Source: CAD feature listing. Evaluate the final solid. Frame: model axes, mm. A direction names the side the tool comes from. Give positions to 0.01 mm unless a question says otherwise; leave off trailing zeros. Loops run counter-clockwise (first coordinate to the right, second up) from the corner with the lowest first, then second, coordinate; pieces in that order, holes last.
```python
from build123d import *

# Parameters (mm, degrees)
SKETCH1_R                = 2.1844
BOSS_EXTRUDE1_DEPTH      = 2
SKETCH1_3_W              = 47.380920583
SKETCH1_3_H              = 2
BOSS_EXTRUDE2_DEPTH      = 2
BOSS_EXTRUDE2_DEPTH_BACK = 122.9409
SKETCH2_R                = 3
SKETCH2_W                = 47.380920583
SKETCH2_H                = 2
SKETCH2_R_2              = 2.5
BOSS_EXTRUDE3_DEPTH      = 2
SKETCH2_3_R              = 3
SKETCH2_3_R_2            = 2.5
BOSS_EXTRUDE4_DEPTH      = 1
SKETCH2_4_R              = 2.5
BOSS_EXTRUDE5_DEPTH      = 6
CHAMFER1_SIZE            = 0.5
SKETCH3_R                = 4.5
SKETCH3_R_2              = 1
CUT_EXTRUDE1_DEPTH       = 10
BOSS_EXTRUDE6_DEPTH      = 8.99804


with BuildPart() as part:
    # Sketch1 → Boss-Extrude1 (new body)
    with BuildSketch(Plane(origin=(0, 0, 0), x_dir=(1, 0, 0), z_dir=(0, 1, 0))):
        with BuildLine():
            ThreePointArc((14.738721003, 0), (0, 13.282171548), (-14.738721003, 0))
            Line((-14.738721003, 0), (-23.700563463, -94.809011723))
            Line((-23.700563463, -94.809011723), (23.68035712, -94.809011723))
            Line((23.68035712, -94.809011723), (14.738721003, 0))
        make_face()
        with BuildLine():
            ThreePointArc((-6.524844791, -45.395600002), (-5.978744791, -41.766355211), (-2.8956, -43.757300002))
            ThreePointArc((-2.8956, -43.757300002), (-3.089055209, -44.656044793), (-3.635155209, -45.395600002))
            ThreePointArc((-3.635155209, -45.395600002), (-5.08, -45.941700002), (-6.524844791, -45.395600002))
        make_face(mode=Mode.SUBTRACT)
        with Locations((5.08, -43.757300002)):
            Circle(SKETCH1_R, mode=Mode.SUBTRACT)
        with Locations((-5.08, 3.740699998)):
            Circle(SKETCH1_R, mode=Mode.SUBTRACT)
        Polygon((-10, 0), (0, 0), (10, 0), (10, -40), (-10, -40), align=None, mode=Mode.SUBTRACT)
        with Locations((5.08, 3.740699998)):
            Circle(SKETCH1_R, mode=Mode.SUBTRACT)
    extrude(amount=BOSS_EXTRUDE1_DEPTH)

    # Sketch1_3 → Boss-Extrude2 (add, two sides)
    with BuildSketch(Plane(origin=(0, 0, 0), x_dir=(1, 0, 0), z_dir=(0, 1, 0))) as boss_extrude2_sk:
        with Locations((-0.010103172, -95.809011723)):
            Rectangle(SKETCH1_3_W, SKETCH1_3_H)
    extrude(amount=BOSS_EXTRUDE2_DEPTH)
    extrude(boss_extrude2_sk.sketch, amount=-BOSS_EXTRUDE2_DEPTH_BACK)

    # Sketch2 → Boss-Extrude3 (add)
    with BuildSketch(Plane.XZ.offset(122.9409)):
        with BuildLine():
            ThreePointArc((14.71851466, 0), (-0.020206343, -13.282171548), (-14.758927346, 0))
            Line((-14.758927346, 0), (-23.700563463, 94.809011723))
            Line((-23.700563463, 94.809011723), (23.68035712, 94.809011723))
            Line((23.68035712, 94.809011723), (14.71851466, 0))
        make_face()
        with Locations((0, 9.721300002)):
            Circle(SKETCH2_R, mode=Mode.SUBTRACT)
        with Locations((-0.010103172, 95.809011723)):
            Rectangle(SKETCH2_W, SKETCH2_H)
        with Locations((0, 9.721300002)):
            Circle(SKETCH2_R)
        with Locations((0, 9.721300002)):
            Circle(SKETCH2_R_2, mode=Mode.SUBTRACT)
        with Locations((0, 9.721300002)):
            Circle(SKETCH2_R_2)
    extrude(amount=BOSS_EXTRUDE3_DEPTH)

    # Sketch2_3 → Boss-Extrude4 (add)
    with BuildSketch(Plane.XZ.offset(122.9409)):
        with Locations((0, 9.721300002)):
            Circle(SKETCH2_3_R)
        with Locations((0, 9.721300002)):
            Circle(SKETCH2_3_R_2, mode=Mode.SUBTRACT)
    extrude(amount=-BOSS_EXTRUDE4_DEPTH)

    # Sketch2_4 → Boss-Extrude5 (add)
    with BuildSketch(Plane.XZ.offset(122.9409)):
        with Locations((0, 9.721300002)):
            Circle(SKETCH2_4_R)
    extrude(amount=-BOSS_EXTRUDE5_DEPTH)

    # Chamfer1
    chamfer1_edges = [part.edges().sort_by_distance(p)[0] for p in [
        (-2.5, -116.9409, 9.721300002),
    ]]
    chamfer(chamfer1_edges, length=CHAMFER1_SIZE)

    # Sketch3 → Cut-Extrude1 (cut)
    with BuildSketch(Plane(origin=(0, 0, 94.809011723), x_dir=(-1, 0, 0), z_dir=(0, 0, -1))):
        with Locations((0.010103172, -61.47045)):
            Circle(SKETCH3_R)
        with Locations((6.260103172, -61.47045)):
            Circle(SKETCH3_R_2)
        with Locations((0.010103172, -67.72045)):
            Circle(SKETCH3_R_2)
        with Locations((-6.239896828, -61.47045)):
            Circle(SKETCH3_R_2)
        with Locations((0.010103172, -55.22045)):
            Circle(SKETCH3_R_2)
    extrude(amount=-CUT_EXTRUDE1_DEPTH, mode=Mode.SUBTRACT)

    # Sketch4 → Boss-Extrude6 (add)
    with BuildSketch(Plane.XY.offset(96.809011723)):
        with BuildLine():
            ThreePointArc((-23.700563463, -98.548234335), (-0.010103172, -105.47045), (23.68035712, -98.548234335))
            Line((23.68035712, -98.548234335), (23.68035712, -96.151310589))
            ThreePointArc((23.68035712, -96.151310589), (-0.010103172, -103.47045), (-23.700563463, -96.151310589))
            Line((-23.700563463, -96.151310589), (-23.700563463, -98.548234335))
        make_face()
        with BuildLine():
            ThreePointArc((-23.700563463, -26.789589411), (-0.010103172, -19.47045), (23.68035712, -26.789589411))
            Line((23.68035712, -26.789589411), (23.68035712, -24.392665665))
            ThreePointArc((23.68035712, -24.392665665), (-0.010103172, -17.47045), (-23.700563463, -24.392665665))
            Line((-23.700563463, -24.392665665), (-23.700563463, -26.789589411))
        make_face()
    extrude(amount=BOSS_EXTRUDE6_DEPTH)


solid = part.part
```
(1) Section A-A, the plane z = 68.5. Return the cut outline in (x, y), then the cut area to 3 significant figures.
A:
outline: (-21.22, -124.94) - (21.19, -124.94) - (21.19, -122.94) - (-21.22, -122.94) - close; (-21.21, 0) - (21.2, 0) - (21.2, 2) - (-21.21, 2) - close
area: 170 mm2
(2) Ray query, line 1 along Y through (x, z) = (-16.5, 86); line 2 along Z through (x, y) = (5.08, 1.3); line 3 along Y through (x, z) = (-1.5, 2). Return the intervals inside material, ascending.
A:
line 1: y = -124.94 to -122.94, 0 to 2
line 2: z = -12.38 to -5.93, -1.56 to 0, 40 to 41.57, 45.94 to 96.81
line 3: y = -124.94 to -122.94
(3) Mould query, pull axis X, two halves, no side actions, for faces 1 (the cylindrical face through (-0.33, -119.72, 12.2)), 2 (the cylindrical face through (0.34, -103.47, 101.25)), 3 (the flat face through (0, 2, 53)). Classes: pulls with the +X half, pulls with the -X half, needs draft (parallel to the pull), parting line crosses it, or undercut.
A:
face 1: parting line crosses it
face 2: undercut
face 3: needs draft
(4) Section C-C, the plane y = -35.5. Return the cut outline in (x, z), then the cut area to 3 significant figures.
A:
outline: (-23.7, 94.81) - (23.68, 94.81) - (23.68, 96.81) - (-23.7, 96.81) - close
area: 94.8 mm2
(5) Section B-B, the plane x = 12. Return the cut outline in (y, z), then the cut area to 3 significant figures.
A:
outline: (-124.94, -7.13) - (-122.94, -7.13) - (-122.94, 94.81) - (0, 94.81) - (0, -7.16) - (2, -7.16) - (2, 96.81) - (-19.14, 96.81) - (-19.14, 105.81) - (-21.22, 105.81) - (-21.22, 96.81) - (-101.72, 96.81) - (-101.72, 105.81) - (-103.8, 105.81) - (-103.8, 96.81) - (-124.94, 96.81) - close
area: 699 mm2
(6) Reachability of faces 4 (the flat face through (0, 0, 52)), 5 (the cylindrical face through (-0.36, -19.47, 101.25)), 6 (the cylindrical face through (-5.554, 0.986, -1.608)), 7 (the flat face through (19.272, 0.986, 48.068)), 8 (the flat face through (-19.167, -123.927, 46.741)) from +Z, -Z, +X, -X, +Y, -Y: full face, straight path, thin tool, end or side. Return the list, or none.
A:
face 4: -Z, +X, -X
face 5: +Z
face 6: +Y
face 7: -Z, +X, +Y, -Y
face 8: -Z, -X, +Y, -Y
(7) First-contact query: pin 1 (3 mm diameter, centred on x = -0.01, y = -67.72, fed in from +Z); pin 2 (12 mm diameter, centred on y = -29.5, z = 93, fed in from +X); pin 3 (1.2 mm diameter, centred on x = -6.26, y = -61.47, fed in from -Z); pin 4 (1 mm diameter, centred on y = 1, z = 25, fed in from +X). Flat tips, straight axial feed; report the tip coordinate or a pass-through.
A:
pin 1: stops at z = 96.81
pin 2: stops at x = 23.68
pin 3: passes through
pin 4: stops at x = 17.14
